```python
from build123d import *

# Parameters (mm, degrees)
SKETCH_1_W          = 200
SKETCH_1_H          = 120
SKETCH_1_R          = 10
SKETCH_1_W_2        = 15
SKETCH_1_H_2        = 10
EXTRUDE_1_DEPTH     = 10
SKETCH_2_W          = 200
SKETCH_2_H          = 120
SKETCH_2_W_2        = 180
SKETCH_2_H_2        = 100
EXTRUDE_2_DEPTH     = 116
SKETCH_4_W          = 200
SKETCH_4_H          = 120
EXTRUDE_3_DEPTH     = 10
SKETCH_6_W          = 200
SKETCH_6_H          = 20
CUT_EXTRUDE_1_DEPTH = 126
SKETCH_7_W          = 200
SKETCH_7_H          = 126
EXTRUDE_4_DEPTH     = 5
SKETCH_8_W          = 200
SKETCH_8_H          = 126
EXTRUDE_5_DEPTH     = 5
SKETCH_9_R          = 8
EXTRUDE_6_DEPTH     = 20
SKETCH_10_R         = 5
EXTRUDE_7_DEPTH     = 5
EXTRUDE_START       = 5
SKETCH_11_R         = 5
EXTRUDE_8_DEPTH     = 5


with BuildPart() as part:
    # 草图1 → 凸台-拉伸1 (new body)
    with BuildSketch(Plane(origin=(0, 0, 0), x_dir=(1, 0, 0), z_dir=(0, 1, 0))):
        Rectangle(SKETCH_1_W, SKETCH_1_H)
        with Locations(Location((0, 25, 0), (0, 0, 270))):
            Circle(SKETCH_1_R, mode=Mode.SUBTRACT)
        with Locations(Location((0, -25, 0), (0, 0, 90))):
            Circle(SKETCH_1_R, mode=Mode.SUBTRACT)
        with Locations((-70.5, 45)):
            Rectangle(SKETCH_1_W_2, SKETCH_1_H_2, mode=Mode.SUBTRACT)
        with Locations((-70.5, -45)):
            Rectangle(SKETCH_1_W_2, SKETCH_1_H_2, mode=Mode.SUBTRACT)
    extrude(amount=EXTRUDE_1_DEPTH)

    # 草图2 → 凸台-拉伸2 (add)
    with BuildSketch(Plane.XZ):
        Rectangle(SKETCH_2_W, SKETCH_2_H)
        Rectangle(SKETCH_2_W_2, SKETCH_2_H_2, mode=Mode.SUBTRACT)
    extrude(amount=EXTRUDE_2_DEPTH)

    # 草图4 → 凸台-拉伸3 (add)
    with BuildSketch(Plane.XZ.offset(116)):
        Rectangle(SKETCH_4_W, SKETCH_4_H)
    extrude(amount=EXTRUDE_3_DEPTH)

    # 草图6 → 切除-拉伸1 (cut)
    with BuildSketch(Plane.XZ.offset(126)):
        Rectangle(SKETCH_6_W, SKETCH_6_H)
    extrude(amount=-CUT_EXTRUDE_1_DEPTH, mode=Mode.SUBTRACT)

    # 草图7 → 凸台-拉伸4 (add)
    with BuildSketch(Plane(origin=(0, 0, 10), x_dir=(-1, 0, 0), z_dir=(0, 0, -1))):
        with Locations((0, -63)):
            Rectangle(SKETCH_7_W, SKETCH_7_H)
    extrude(amount=-EXTRUDE_4_DEPTH)

    # 草图8 → 凸台-拉伸5 (add)
    with BuildSketch(Plane.XY.offset(-10)):
        with Locations((0, -63)):
            Rectangle(SKETCH_8_W, SKETCH_8_H)
    extrude(amount=-EXTRUDE_5_DEPTH)

    # 草图9 → 凸台-拉伸6 (add)
    with BuildSketch(Plane.XY.offset(-10)):
        with Locations(Location((0, -20, 0), (0, 0, 180))):
            Circle(SKETCH_9_R)
    extrude(amount=EXTRUDE_6_DEPTH)

    # 草图10 → 凸台-拉伸7 (add)
    with BuildSketch(Plane.XY.offset(60)):
        with Locations(Location((0, -20, 0), (0, 0, 180))):
            Circle(SKETCH_10_R)
    extrude(amount=EXTRUDE_7_DEPTH)

    # 草图11 → 凸台-拉伸8 (add)
    with BuildSketch(Plane(origin=(0, 0, -60), x_dir=(-1, 0, 0), z_dir=(0, 0, -1)).offset(EXTRUDE_START)):
        with Locations((0, -20)):
            Circle(SKETCH_11_R)
    extrude(amount=-EXTRUDE_8_DEPTH)


solid = part.part
```
Design review of the part built by this model. Coordinates are the model's own, in mm. A direction names the side the tool comes from. Give positions to 0.01 mm unless a question says otherwise; leave off trailing zeros. Order: outer loops, then holes, each group sorted by start corner. A loop starts at its lowest first (then second) coordinate and runs counter-clockwise, first axis right, second up. Notation, with made-up numbers: (57, 49.25) - (78, 49.25) arc R30 ccw to (78, 81.25) - close; hole circle Ø7 at (-15.75, 67). An arc over 180 degrees is marked (long way). Use a Markdown table: item, result. Add a question column.
(1) Wall thickness on probe 1 along Z at (x, y) = (-21.5, -80); probe 2 along X at (y, z) = (-61, -31); probe 3 along Y at (x, z) = (31.5, 40.5): over which ranges is each line inside the solid? List them lowest first. Write a range as [from, to].
(2) Add section B-B on x = -30.5. Give the boundary of the cut face in (y, z), then the cut area to 3 significant figures.
(3) Add section C-C on y = -20. Give the boundary of the cut face in (x, z).
(4) Add section A-A on y = -88.5. Give the boundary of the cut face in (x, z).
(5) Mouldability with a two-part tool opening along X and no side actions: class faces 4 (the face through (1.08, -24.88, -62.54)), 5 (the face through (-1, -116, -32)), 6 (the face through (-1, -64, -10)) as +X half, -X half, draft (parallel to the pull), parting line (faces both ways), or undercut.
(6) Machinability: for faces 1 (the face through (-78, 5, -45)), 2 (the face through (-1, -57, -15)), 3 (the face through (-1, -126, -35)), which of the approach directions +Z, -Z, +X, -X, +Y, -Y give a long, thin tool a straight path to every point of the face, cutting with its end or side? Answer none if there is none.
(7) Add section D-D on z = -47.5. Give the boundary of the cut face in (x, y).
(8) Clearance check with flat-ended pins moving along their axes: P1, Ø2, axis at x = -66, y = -4, coming from the -Z side; P2, Ø6, axis at x = 48, z = -3, coming from the -Y side. State where each tip first meets the part, or that it passes through.
Report:
| question | item | result |
|---|---|---|
| 1 | probe 1 | z = [-60, -50], [-15, -10], [10, 15], [50, 60] |
| 1 | probe 2 | x = [-100, -90], [90, 100] |
| 1 | probe 3 | y = [-126, -116], [0, 10] |
| 2 | outline | (-126, -60) - (10, -60) - (10, 60) - (-126, 60) - (-126, 10) - (0, 10) - (0, -10) - (-126, -10) - close; hole (-116, -50) - (0, -50) - (0, -15) - (-116, -15) - close; hole (-116, 15) - (0, 15) - (0, 50) - (-116, 50) - close |
| 2 | area | 5,680 mm² |
| 3 | outline | (-100, -60) - (-5, -60) - (-5, -65) - (5, -65) - (5, -60) - (100, -60) - (100, -10) - (8, -10) - (8, 10) - (100, 10) - (100, 60) - (5, 60) - (5, 65) - (-5, 65) - (-5, 60) - (-100, 60) - (-100, 10) - (-8, 10) - (-8, -10) - (-100, -10) - close; hole (-90, -50) - (90, -50) - (90, -15) - (-90, -15) - close; hole (-90, 15) - (90, 15) - (90, 50) - (-90, 50) - close |
| 4 | outline | (-100, -60) - (100, -60) - (100, -10) - (-100, -10) - close; (-100, 10) - (100, 10) - (100, 60) - (-100, 60) - close; hole (-90, -50) - (90, -50) - (90, -15) - (-90, -15) - close; hole (-90, 15) - (90, 15) - (90, 50) - (-90, 50) - close |
| 5 | face 4 | parting line |
| 5 | face 5 | undercut |
| 5 | face 6 | draft |
| 6 | face 1 | +Y |
| 6 | face 2 | none |
| 6 | face 3 | +Z, -Z, +X, -X, -Y |
| 7 | outline | (-100, -126) - (100, -126) - (100, 10) - (-63, 10) - (-63, 0) - (90, 0) - (90, -116) - (-90, -116) - (-90, 0) - (-78, 0) - (-78, 10) - (-100, 10) - close |
| 8 | P1 | stops at z = -60 |
| 8 | P2 | stops at y = 0 |
